Geometry: final body of the model. Coordinates: model frame, mm. Face numbers are marked on the shaded views. A direction names the side the tool comes from. Round coordinates to 2 decimals unless told otherwise and drop trailing zeros. Order: outer loops, then holes, each group sorted by start corner. A loop starts at its lowest first (then second) coordinate and runs counter-clockwise, first axis right, second up. Notation, with made-up numbers: M 24.5,-26 L 66.5,-26 A29 ccw 66.5,3 Z; hole C 8,-27.5 d11. An arc over 180 degrees is marked long. Put each result on its own line as item: value. Start each with the question number.
1) Section A-A, the plane x = 18. Return loops of the section in (y, z), then the cut area to 3 significant figures.
2) Section B-B, the plane y = 38. Return loops of the section in (x, z).
3) Section D-D, the plane z = -3. Return loops of the section in (x, y).
4) Access query for the marked faces 1, 2 and 3. Directions: +Z, -Z, +X, -X, +Y, -Y. A direction counts if a zero-diameter tool reaches every point of the face in a straight line with its end or side. Return the directions, or none.
5) First-contact query: P1, Ø5.5, axis at y = 1.5, z = -12, coming from the +X side; P2, Ø16.5, axis at x = 20.5, y = 45.5, coming from the -Z side; P3, Ø8, axis at x = 1, z = 18, coming from the -Y side; P4, Ø12, axis at y = 12, z = 10, coming from the -X side. Flat tips, straight axial feed; report the tip coordinate or a pass-through.
6) Material intervals for probe 1 along X at (y, z) = (3, -10); probe 2 along Z at (x, y) = (18, 48.5); probe 3 along X at (y, z) = (38, 8), sorted ascending. Write a range as [from, to].
7) Section C-C, the plane x = 30. Return loops of the section in (y, z), then the cut area to 3 significant figures.
8) Draft query along Y for the marked faces 4, 5, 6 and 7. Return one class per face: pulls with the +Y half, pulls with the -Y half, needs draft (parallel to the pull), parting line crosses it, or undercut.
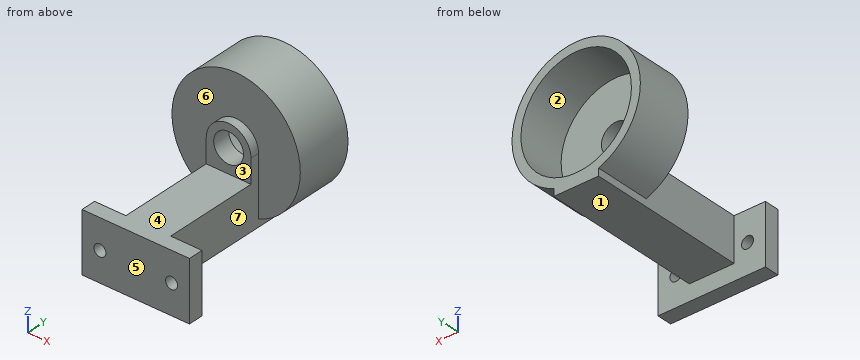
from build123d import *

# Parameters (mm, degrees)
ESQUISSE1_W             = 36
ESQUISSE1_H             = 20
BOSS_EXTRU_1_DEPTH      = 5
ESQUISSE2_W             = 15
ESQUISSE2_H             = 10.591208458
ESQUISSE2_H_2           = 4
BOSS_EXTRU_2_DEPTH      = 32
ESQUISSE3_R             = 5
BOSS_EXTRU_3_DEPTH      = 6
ESQUISSE4_R             = 21.5
ESQUISSE4_R_2           = 18.5
BOSS_EXTRU_4_DEPTH      = 16
BOSS_EXTRU_5_START      = -3
ESQUISSE5_R             = 21.5
ESQUISSE5_R_2           = 7.5
BOSS_EXTRU_5_DEPTH      = 3
ESQUISSE6_W             = 15
ESQUISSE6_H             = 3.413220749
BOSS_EXTRU_6_DEPTH      = 16
ESQUISSE8_R             = 2
ENL_V_MAT_EXTRU_1_DEPTH = 16


with BuildPart() as part:
    # Esquisse1 → Boss.-Extru.1 (new body)
    with BuildSketch(Plane(origin=(0, 0, 0), x_dir=(1, 0, 0), z_dir=(0, 1, 0))):
        with Locations((18, 10)):
            Rectangle(ESQUISSE1_W, ESQUISSE1_H)
    extrude(amount=BOSS_EXTRU_1_DEPTH)

    # Esquisse2 → Boss.-Extru.2 (add)
    with BuildSketch(Plane(origin=(0, 5, 0), x_dir=(1, 0, 0), z_dir=(0, 1, 0))):
        with Locations((18, 5.295604229)):
            Rectangle(ESQUISSE2_W, ESQUISSE2_H)
        with Locations((18, 12.591208458)):
            Rectangle(ESQUISSE2_W, ESQUISSE2_H_2)
    extrude(amount=BOSS_EXTRU_2_DEPTH)

    # Esquisse3 → Boss.-Extru.3 (add)
    with BuildSketch(Plane(origin=(0, 37, 0), x_dir=(1, 0, 0), z_dir=(0, 1, 0))):
        with BuildLine():
            Line((10.5, 14.591208458), (10.5, -8))
            ThreePointArc((10.5, -8), (18, -15.5), (25.5, -8))
            Line((25.5, -8), (25.5, 14.591208458))
            Line((25.5, 14.591208458), (10.5, 14.591208458))
        make_face()
        with Locations(Location((18, -8, 0), (0, 0, 270))):
            Circle(ESQUISSE3_R, mode=Mode.SUBTRACT)
    extrude(amount=BOSS_EXTRU_3_DEPTH)

    # Esquisse4 → Boss.-Extru.4 (add)
    with BuildSketch(Plane(origin=(0, 43, 0), x_dir=(1, 0, 0), z_dir=(0, 1, 0))):
        with Locations(Location((18, -8, 0), (0, 0, 69.583789871))):
            Circle(ESQUISSE4_R)
        with Locations(Location((18, -8, 0), (0, 0, 66.083465578))):
            Circle(ESQUISSE4_R_2, mode=Mode.SUBTRACT)
    extrude(amount=BOSS_EXTRU_4_DEPTH)

    # Esquisse5 → Boss.-Extru.5 (add)
    with BuildSketch(Plane(origin=(0, 43, 0), x_dir=(1, 0, 0), z_dir=(0, 1, 0)).offset(BOSS_EXTRU_5_START)):
        with Locations(Location((18, -8, 0), (0, 0, 69.583789871))):
            Circle(ESQUISSE5_R)
        with Locations((18, -8)):
            Circle(ESQUISSE5_R_2, mode=Mode.SUBTRACT)
    extrude(amount=BOSS_EXTRU_5_DEPTH)

    # Esquisse6 → Boss.-Extru.6 (add)
    with BuildSketch(Plane(origin=(0, 43, 0), x_dir=(1, 0, 0), z_dir=(0, 1, 0))):
        with Locations((18, 12.884598084)):
            Rectangle(ESQUISSE6_W, ESQUISSE6_H)
    extrude(amount=BOSS_EXTRU_6_DEPTH)

    # Esquisse8 → Enlèv. mat.-Extru.1 (cut)
    with BuildSketch(Plane.XZ):
        with Locations(Location((6, -10, 0), (0, 0, 270))):
            Circle(ESQUISSE8_R)
        with Locations(Location((30, -10, 0), (0, 0, 270))):
            Circle(ESQUISSE8_R)
    extrude(amount=-ENL_V_MAT_EXTRU_1_DEPTH, mode=Mode.SUBTRACT)


solid = part.part
Result sheet:
1. outline: M 0,-20 L 5,-20 L 5,-14.59 L 59,-14.59 L 59,-10.5 L 43,-10.5 L 43,3 L 37,3 L 37,0 L 0,0 Z; M 37,13 L 43,13 L 43,26.5 L 59,26.5 L 59,29.5 L 40,29.5 L 40,15.5 L 37,15.5 Z
1. area: 843 mm2
2. outline: M 10.5,-14.59 L 25.5,-14.59 L 25.5,8 A7.5 ccw 10.5,8 Z; hole C 18,8 d10
3. outline: M -0.47,40 L 10.5,40 L 10.5,5 L 0,5 L 0,0 L 36,0 L 36,5 L 25.5,5 L 25.5,40 L 36.47,40 L 36.47,59 L 32.87,59 L 32.87,43 L 3.13,43 L 3.13,59 L -0.47,59 Z
4. face 1: -Z, +X, -X, +Y
4. face 2: +Y
4. face 3: +Z, +X, -X, -Y
5. P1: stops at x = 36
5. P2: stops at z = -14.59
5. P3: stops at y = 40
5. P4: passes through
6. probe 1: x = [0, 4], [8, 28], [32, 36]
6. probe 2: z = [-14.59, -10.5], [26.5, 29.5]
6. probe 3: x = [10.5, 13], [23, 25.5]
7. outline: M 0,-20 L 5,-20 L 5,-12 L 0,-12 Z; M 0,-8 L 5,-8 L 5,0 L 0,0 Z; M 40,-9.84 L 59,-9.84 L 59,-6.08 L 43,-6.08 L 43,22.08 L 59,22.08 L 59,25.84 L 40,25.84 Z
7. area: 307 mm2
8. face 4: needs draft
8. face 5: pulls with the -Y half
8. face 6: undercut
8. face 7: undercut
